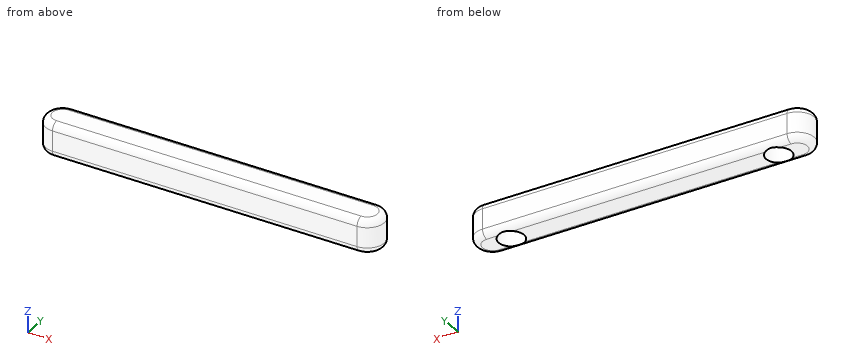
```python
from build123d import *

# Parameters (mm, degrees)
BOSS_EXTRUDE1_DEPTH = 12.7
SKETCH2_R           = 4.7625
CUT_EXTRUDE1_DEPTH  = 6.35
FILLET1_R           = 2.54


with BuildPart() as part:
    # Sketch1 → Boss-Extrude1 (new body)
    with BuildSketch(Plane.XY):
        with BuildLine():
            Line((0, 0), (114.3, 0))
            ThreePointArc((114.3, 0), (120.65, -6.35), (114.3, -12.7))
            Line((114.3, -12.7), (0, -12.7))
            ThreePointArc((0, -12.7), (-6.35, -6.35), (0, 0))
        make_face()
    extrude(amount=-BOSS_EXTRUDE1_DEPTH)

    # Sketch2 → Cut-Extrude1 (cut)
    with BuildSketch(Plane(origin=(0, 0, -12.7), x_dir=(-1, 0, 0), z_dir=(0, 0, -1))):
        with Locations((-6.985, -6.35)):
            Circle(SKETCH2_R)
        with Locations((-107.315, -6.35)):
            Circle(SKETCH2_R)
    extrude(amount=-CUT_EXTRUDE1_DEPTH, mode=Mode.SUBTRACT)

    # Fillet1
    # the kernel refuses this fillet: 2.54 mm, written as the material it takes off along each edge
    with BuildSketch(Plane(origin=(114.3, -6.35, -12.7), x_dir=(0, 1, 0), z_dir=(-1, 0, 0))) as fillet1_piece_1:
        with BuildLine():
            CenterArc((6.35 - FILLET1_R, -FILLET1_R), FILLET1_R, 0, 90)
            Line((6.35 - FILLET1_R, 0), (6.35, 0))
            Line((6.35, 0), (6.35, -FILLET1_R))
        make_face()
    revolve(axis=Axis((114.3, -6.35, -12.7), (0, 0, -1)), revolution_arc=180, mode=Mode.SUBTRACT)
    with BuildSketch(Plane(origin=(0, 0, -12.7), x_dir=(0, -1, 0), z_dir=(1, 0, 0)), Plane(origin=(114.3, -12.7, 0), x_dir=(0, 0, -1), z_dir=(-1, 0, 0))) as fillet1_piece_2:
        with BuildLine():
            CenterArc((FILLET1_R, -FILLET1_R), FILLET1_R, 90, 90)
            Line((0, -FILLET1_R), (0, 0))
            Line((0, 0), (FILLET1_R, 0))
        make_face()
    extrude(amount=114.3, mode=Mode.SUBTRACT)
    with BuildSketch(Plane(origin=(0, -6.35, -12.7), x_dir=(0, -1, 0), z_dir=(1, 0, 0))) as fillet1_piece_3:
        with BuildLine():
            CenterArc((6.35 - FILLET1_R, -FILLET1_R), FILLET1_R, 0, 90)
            Line((6.35 - FILLET1_R, 0), (6.35, 0))
            Line((6.35, 0), (6.35, -FILLET1_R))
        make_face()
    revolve(axis=Axis((0, -6.35, -12.7), (0, 0, -1)), revolution_arc=180, mode=Mode.SUBTRACT)
    with BuildSketch(Plane(origin=(0, 0, 0), x_dir=(0, -1, 0), z_dir=(1, 0, 0)), Plane(origin=(114.3, -12.7, -12.7), x_dir=(0, 0, 1), z_dir=(-1, 0, 0))) as fillet1_piece_4:
        with BuildLine():
            CenterArc((FILLET1_R, FILLET1_R), FILLET1_R, 180, 90)
            Line((0, FILLET1_R), (0, 0))
            Line((0, 0), (FILLET1_R, 0))
        make_face()
    extrude(amount=114.3, mode=Mode.SUBTRACT)
    with BuildSketch(Plane(origin=(114.3, -6.35, 0), x_dir=(0, 1, 0), z_dir=(-1, 0, 0))) as fillet1_piece_5:
        with BuildLine():
            CenterArc((6.35 - FILLET1_R, FILLET1_R), FILLET1_R, 270, 90)
            Line((6.35 - FILLET1_R, 0), (6.35, 0))
            Line((6.35, 0), (6.35, FILLET1_R))
        make_face()
    revolve(axis=Axis((114.3, -6.35, 0), (0, 0, -1)), revolution_arc=180, mode=Mode.SUBTRACT)
    with BuildSketch(Plane(origin=(0, -6.35, 0), x_dir=(0, -1, 0), z_dir=(1, 0, 0))) as fillet1_piece_6:
        with BuildLine():
            CenterArc((6.35 - FILLET1_R, FILLET1_R), FILLET1_R, 270, 90)
            Line((6.35 - FILLET1_R, 0), (6.35, 0))
            Line((6.35, 0), (6.35, FILLET1_R))
        make_face()
    revolve(axis=Axis((0, -6.35, 0), (0, 0, -1)), revolution_arc=180, mode=Mode.SUBTRACT)


solid = part.part
```
Model file for the job. Use its own axes, mm. Coordinates: 2 decimals unless noted, no trailing zeros. Loops run counter-clockwise (first coordinate to the right, second up) from the corner with the lowest first, then second, coordinate; pieces in that order, holes last. Notation, with made-up numbers: (59, -1) - (64, -1) arc R16 ccw to (64, 4) - close; hole circle Ø6 at (-19.75, 65.25). An arc over 180 degrees is marked (long way). Write item = value, one per line. Start each with the question number.
Item 1: Saw through at A-A, the plane z = -8.25. State how many separate pieces and enclosed holes the cut face has, then the cut area to 3 significant figures.
Item 2: Saw through at C-C, the plane x = 8.5. List the corners of the cut face in (y, z), then the cut area to 3 significant figures.
Item 3: Wall check: probe 1 along X at (y, z) = (-6.35, -8.75); probe 2 along X at (y, z) = (-5.75, -10); probe 3 along Y at (x, z) = (10.5, -8.25). Give the ranges that are in metal, low to high. Write a range as [from, to].
Item 4: Saw through at B-B, the plane y = -6.35. List the corners of the cut face in (x, z).
Item 5: Saw through at D-D, the plane x = 83. List the corners of the cut face in (y, z), then the cut area to 3 significant figures.
Answers:
q1.separate_pieces = 1
q1.enclosed_holes = 2
q1.area = 1,440 mm2
q2.outline = (-12.7, -10.16) arc R2.54 ccw to (-10.87, -12.6) - (-10.87, -6.35) - (-1.83, -6.35) - (-1.83, -12.6) arc R2.54 ccw to (0, -10.16) - (0, -2.54) arc R2.54 ccw to (-2.54, 0) - (-10.16, 0) arc R2.54 ccw to (-12.7, -2.54) - close
q2.area = 98.5 mm2
q3.probe_1 = [-6.35, 2.22], [11.75, 102.55], [112.08, 120.65]
q3.probe_2 = [-6.32, 2.26], [11.71, 102.59], [112.04, 120.62]
q3.probe_3 = [-12.7, -9.56], [-3.14, 0]
q4.outline = (-6.35, -10.16) arc R2.54 ccw to (-3.81, -12.7) - (2.22, -12.7) - (2.22, -6.35) - (11.75, -6.35) - (11.75, -12.7) - (102.55, -12.7) - (102.55, -6.35) - (112.08, -6.35) - (112.08, -12.7) - (118.11, -12.7) arc R2.54 ccw to (120.65, -10.16) - (120.65, -2.54) arc R2.54 ccw to (118.11, 0) - (-3.81, 0) arc R2.54 ccw to (-6.35, -2.54) - close
q5.outline = (-12.7, -10.16) arc R2.54 ccw to (-10.16, -12.7) - (-2.54, -12.7) arc R2.54 ccw to (0, -10.16) - (0, -2.54) arc R2.54 ccw to (-2.54, 0) - (-10.16, 0) arc R2.54 ccw to (-12.7, -2.54) - close
q5.area = 156 mm2
